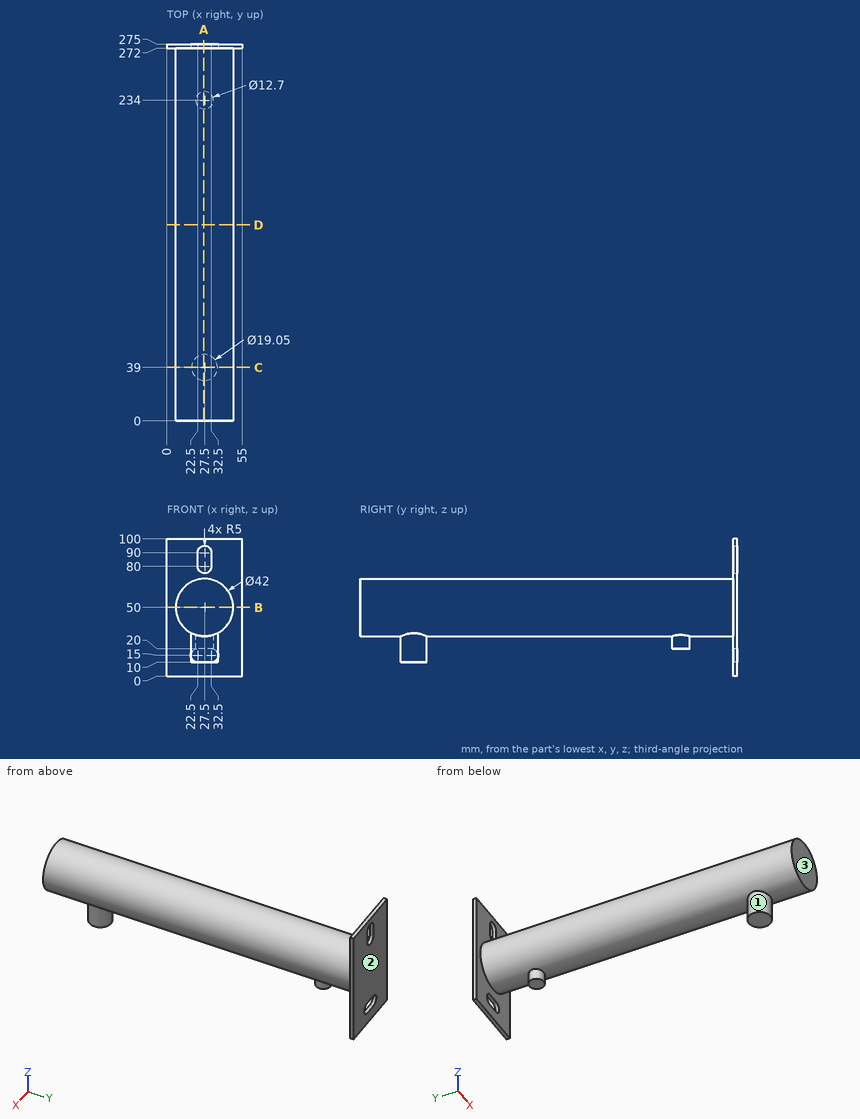
The figure shows three views and two pictorial views of one solid part (mm, origin at its lowest corner). Answer the questions. Coordinates: 2 decimals unless noted, no trailing zeros. Write each loop counter-clockwise with the first axis right and the second up, starting at its lowest first coordinate (ties: lowest second). Pieces come first, ordered by that corner, then holes. Notation, with made-up numbers: (48, 64) -> (61, 64) arc R26 cw to (61, 83) -> close; hole circle Ø8 at (9.25, -33.5). An arc over 180 degrees is marked (long way). Return JSON: item names as keys, results as strings.
1. A cutting plane is placed at A-A (x = 27). Determine the outline of the cut face in (y, z).
Found:
{"outline": "(0, 29.01) -> (29.49, 29.01) -> (29.49, 10) -> (48.51, 10) -> (48.51, 29.01) -> (227.67, 29.01) -> (227.67, 20) -> (240.33, 20) -> (240.33, 29.01) -> (272, 29.01) -> (272, 20) -> (275, 20) -> (275, 75.03) -> (272, 75.03) -> (272, 70.99) -> (0, 70.99) -> close; (272, 0) -> (275, 0) -> (275, 10) -> (272, 10) -> close; (272, 94.97) -> (275, 94.97) -> (275, 100) -> (272, 100) -> close"}
2. Find the intervals of material crossed by line 1 along Z through (x, y) = (26, 113); line 2 along Y through (x, z) = (6.5, 76.5); line 3 along X through (y, z) = (145, 48.5), in increasing order. Write a range as from..to.
Found:
{"line 1": "29.05..70.95", "line 2": "272..275", "line 3": "6.55..48.45"}
3. Each of these flat-tipped pins is pushed along its axis until it touches: P1, Ø9.5, axis at x = 25, y = 37, coming from the -Z side; P2, Ø10, axis at x = 28.5, y = 232.5, coming from the -Z side; P3, Ø8, axis at y = 238.5, z = 45, coming from the +X side. Where does it stop, or does it pass through?
Found:
{"P1": "z = 10", "P2": "z = 20", "P3": "x = 48.48"}
4. A cutting plane is placed at D-D (y = 143). Determine the outline of the cut face in (x, z).
Found:
{"outline": "circle Ø42 at (27.5, 50)"}
5. Determine the mould class of the marked faces 1, 2 and 3 for opening direction Y: pulls with the +Y half, pulls with the -Y half, needs draft (parallel to the pull), parting line crosses it, or undercut.
Found:
{"face 1": "undercut", "face 2": "pulls with the +Y half", "face 3": "pulls with the -Y half"}
6. A cutting plane is placed at B-B (z = 50). Determine the outline of the cut face in (x, y).
Found:
{"outline": "(0, 272) -> (6.5, 272) -> (6.5, 0) -> (48.5, 0) -> (48.5, 272) -> (55, 272) -> (55, 275) -> (0, 275) -> close"}
7. A cutting plane is placed at C-C (y = 39). Determine the outline of the cut face in (x, z) (3 decimals).
Found:
{"outline": "(17.975, 10) -> (37.025, 10) -> (37.025, 31.284) arc R21 ccw (long way) to (17.975, 31.284) -> close"}
